Could you check a few things on this model? Use its own coordinates, in mm. Face numbers are marked on the shaded views. A direction names the side the tool comes from. Round coordinates to 2 decimals unless told otherwise and drop trailing zeros. Loops run counter-clockwise (first coordinate to the right, second up) from the corner with the lowest first, then second, coordinate; pieces in that order, holes last. Notation, with made-up numbers: (-8, 17) -> (30, 17) arc R23 ccw to (30, 53) -> close; hole circle Ø6 at (38.5, -22). An arc over 180 degrees is marked (long way). One line per item, written item: value.
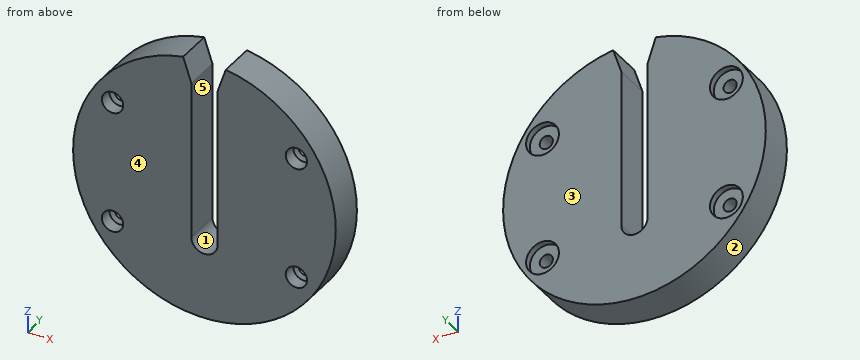
```python
from build123d import *

# Parameters (mm, degrees)
F0_R           = 63.5
F1_DEPTH       = 17.78
F2_D           = 6.35
F2_CBORE_D     = 15.875
F2_CBORE_DEPTH = 3.175
F4_D           = 10.31875
F4_DEPTH       = 6.35
F4_TIP         = 3.1000652563
F6_DEPTH       = 25.4


# Not quite as in the source:
# - a length typed as a fraction of an inch, garbled in the dataset ("3 / 203.2 mm" for 3/8 in), is restored
# - a feature names something its author has since deleted; it is built from what else it names


with BuildPart() as f1:
    # F0 (on Front) → F1 (new body)
    with BuildSketch(Plane.XZ):
        Circle(F0_R)
    extrude(amount=F1_DEPTH)

    # F2 (through all)
    with Locations(Plane(origin=(0, 0, 0), x_dir=(1, 0, 0), z_dir=(0, 1, 0))):
        with Locations((44.45, -29.36875), (-44.45, -29.36875), (-44.45, 29.36875), (44.45, 29.36875)):
            CounterBoreHole(F2_D / 2, F2_CBORE_D / 2, F2_CBORE_DEPTH)

    # F4
    with Locations(Plane.XZ.offset(17.78)):
        with Locations((-44.45, 29.36875), (44.45, 29.36875), (44.45, -29.36875), (-44.45, -29.36875)):
            Hole(F4_D / 2, depth=F4_DEPTH)
            with Locations((0, 0, -(F4_DEPTH + F4_TIP / 2))):  # 118° drill point
                Cone(0, F4_D / 2, F4_TIP, mode=Mode.SUBTRACT)

    # F5 (on face) → F6 (cut)
    with BuildSketch(Plane.XZ.offset(17.78)):
        with BuildLine():
            Line((-10.3124, 62.6570379625), (-6.35, 50.8))
            Line((-6.35, 50.8), (-6.35, -25.4))
            ThreePointArc((-6.35, -25.4), (0, -31.75), (6.35, -25.4))
            Line((6.35, -25.4), (6.35, 50.8))
            Line((6.35, 50.8), (10.3124, 62.6570379625))
            ThreePointArc((10.3124, 62.6570379625), (0, 63.5), (-10.3124, 62.6570379625))
        make_face()
    extrude(amount=-F6_DEPTH, mode=Mode.SUBTRACT)


solid = f1.part
```
(1) Please list where these lines run through material, in increasing order: L1, parallel to Z at x = 44.45, y = -8; L2, parallel to X at y = -14, z = 32.5; L3, parallel to Z at x = 44.45, y = -0.8.
Results below:
L1: z = -45.35 to -32.54, -26.19 to 26.19, 32.54 to 45.35
L2: x = -54.55 to -48.55, -40.35 to -6.35, 6.35 to 40.35, 48.55 to 54.55
L3: z = -45.35 to -37.31, -21.43 to 21.43, 37.31 to 45.35
(2) For pin 1 Ø5 at (x, z) = (-41.5, -27.5) entering from +Y (3 decimals); pin 2 Ø5 at (x, y) = (23.5, -7) entering from +Z; pin 3 Ø2 at (x, z) = (9.5, -33) entering from +Y; pin 4 Ø8.5 at (x, z) = (-44.45, 29.37) entering from -Y, each with a flat end and sliding along its axis, tell me the tip position at first contact or that it passes through.
Results below:
pin 1: stops at y = -3.175
pin 2: stops at z = 59.93
pin 3: stops at y = 0
pin 4: stops at y = -10.88
(3) Imagine slicing it at B-B on y = -16.25. Write out the boundary of the cut face in (x, z).
Results below:
outline: (-10.31, 62.66) arc R63.5 ccw (long way) to (10.31, 62.66) -> (6.35, 50.8) -> (6.35, -25.4) arc R6.35 cw to (-6.35, -25.4) -> (-6.35, 50.8) -> close; hole circle Ø10.32 at (-44.45, -29.37); hole circle Ø10.32 at (-44.45, 29.37); hole circle Ø10.32 at (44.45, -29.37); hole circle Ø10.32 at (44.45, 29.37)
(4) On a 3-axis mill with a long thin cutter (end or side, diameter ignored), from which of +Z, -Z, +X, -X, +Y, -Y can I reach the whole of each face in a straight line? I mean the marked faces 4 and 5. Say none if no direction works.
Results below:
face 4: +Z, -Z, +X, -X, -Y
face 5: +Z, +Y, -Y
(5) Imagine slicing it at A-A on z = 0. Write out the boundary of the cut face in (x, y).
Results below:
outline: (-63.5, -17.78) -> (-6.35, -17.78) -> (-6.35, 0) -> (-63.5, 0) -> close; (6.35, -17.78) -> (63.5, -17.78) -> (63.5, 0) -> (6.35, 0) -> close
(6) Imagine slicing it at C-C on x = -44.45. Write out the boundary of the cut face in (y, z) (3 decimals).
Results below:
outline: (-17.78, -45.348) -> (0, -45.348) -> (0, -37.306) -> (-3.175, -37.306) -> (-3.175, -32.544) -> (-10.238, -32.544) -> (-11.43, -34.528) -> (-17.78, -34.528) -> close; (-17.78, -24.209) -> (-11.43, -24.209) -> (-10.238, -26.194) -> (-3.175, -26.194) -> (-3.175, -21.431) -> (0, -21.431) -> (0, 21.431) -> (-3.175, 21.431) -> (-3.175, 26.194) -> (-10.238, 26.194) -> (-11.43, 24.209) -> (-17.78, 24.209) -> close; (-17.78, 34.528) -> (-11.43, 34.528) -> (-10.238, 32.544) -> (-3.175, 32.544) -> (-3.175, 37.306) -> (0, 37.306) -> (0, 45.348) -> (-17.78, 45.348) -> close
(7) Imagine slicing it at D-D on x = 0. Write out the boundary of the cut face in (y, z), then the cut area to 3 significant figures.
Results below:
outline: (-17.78, -63.5) -> (0, -63.5) -> (0, -31.75) -> (-17.78, -31.75) -> close
area: 565 mm²
(8) We'd pull the mould along X, two halves only. Please class the marked faces 1, 2 and 3: +X half, -X half, draft (parallel to the pull), parting line (faces both ways), or undercut.
Results below:
face 1: undercut
face 2: parting line
face 3: draft
